Autodesk Inventor part; units mm, degrees
ref_plane "YZ Plane" through (0, 0, 0) normal (1, 0, 0) x (0, 1, 0)
ref_plane "XZ Plane" through (0, 0, 0) normal (0, 1, 0) x (-1, 0, 0)
ref_plane "XY Plane" through (0, 0, 0) normal (0, 0, 1) x (1, 0, 0)
sketch "Sketch1" plane through (0, 0, 0) normal (0, 0, 1) x (1, 0, 0)
  line L0 (-31.45, -31.45) -> (31.45, -31.45)
  line L1 (31.45, -31.45) -> (31.45, 31.45)
  line L2 (31.45, 31.45) -> (-31.45, 31.45)
  line L3 (-31.45, 31.45) -> (-31.45, -31.45)
  line L4 (-31.45, -31.45) -> (31.45, 31.45) construction
  line L5 (31.45, -31.45) -> (-31.45, 31.45) construction
  line L6 (-36.45, 36.45) -> (36.45, 36.45)
  line L7 (36.45, 36.45) -> (36.45, -36.45)
  line L8 (36.45, -36.45) -> (-36.45, -36.45)
  line L9 (-36.45, -36.45) -> (-36.45, 36.45)
  point P0 (0, 0)
  dimension "d0" = 62.9
  dimension "d1" = 62.9
  dimension "d2" = 5
extrude "Extrusion1" add sketch "Sketch1" along normal blind 85
sketch "Sketch2" plane through (0, 0, 0) normal (0, 0, -1) x (-1, 0, 0)
  line L0 (31.45, 31.45) -> (-31.45, 31.45)
  line L1 (31.45, -31.45) -> (-31.45, -31.45)
  line L2 (-31.45, -31.45) -> (-31.45, 31.45)
  line L3 (-31.45, 31.45) -> (31.45, 31.45)
  line L4 (31.45, 31.45) -> (31.45, -31.45)
  line L5 (31.45, -31.45) -> (-31.45, 31.45) construction
  line L6 (-31.45, -31.45) -> (31.45, 31.45) construction
  point P0 (0, 0)
  point P1 (31.45, 31.45)
extrude "Extrusion2" add sketch "Sketch2" against normal blind 12.144
sketch "Sketch3" plane through (-36.45, -36.45, 0) normal (-1, 0, 0) x (0, 0, 1)
  line L0 (85, 0) -> (85, 72.9)
  line L1 (85, 0) -> (0, 0)
  line L2 (0, 0) -> (0, 67.9)
  line L3 (0, 67.9) -> (85, 67.9)
  line L4 (85, 67.9) -> (85, 0)
  point P0 (0, 36.45)
extrude "Extrusion3" cut sketch "Sketch3" against normal blind 5
sketch "Sketch4" plane through (0, 0, 0) normal (0, 0, -1) x (-1, 0, 0)
  point P0 (0, 0)
sketch "Sketch5" plane through (-36.45, 31.45, 0) normal (-1, 0, 0) x (0, 0, 1)
  line L0 (0, 5) -> (0, 0)
  line L1 (0, 5) -> (85, 5)
  line L2 (0, 0) -> (85, 0)
  line L3 (85, 5) -> (85, 0)
  point P0 (0, -31.45)
extrude "Extrusion4" cut sketch "Sketch5" against normal blind 5
sketch "Sketch6" plane through (0, 0, 0) normal (0, 0, -1) x (-1, 0, 0)
  circle A0 centre (0, 0) radius 22.545
  dimension "d11" = 45.09
extrude "Extrusion5" cut sketch "Sketch6" against normal blind 5
sketch "Sketch7" plane through (0, 0, 5) normal (0, 0, -1) x (-1, 0, 0)
  circle A0 centre (0, 0) radius 25.4
  dimension "d14" = 50.8
sketch "Sketch8" plane through (0, 0, 12.144) normal (0, 0, 1) x (1, 0, 0)
  point P0 (0, 0)
extrude "Extrusion6" cut sketch "Sketch7" against normal blind 10
sketch "Sketch12" plane through (36.45, 36.45, 85) normal (0, 1, 0) x (1, 0, 0)
  circle A0 centre (-33.8267, 41.9258) radius 12.7
  point P0 (-36.45, 85)
extrude "Extrusion10" cut sketch "Sketch12" along normal blind 5
sketch "Sketch13" plane through (31.45, -31.45, 85) normal (-1, 0, 0) x (0, 0, 1)
  ellipse E0 centre (-53.33, 18.7291) end of major axis (-50.83, 18.7291) minor radius 2.5
  ellipse E1 centre (-27.93, 44.1291) end of major axis (-25.43, 44.1291) minor radius 2.5
  ellipse E2 centre (-53.33, 44.1291) end of major axis (-50.83, 44.1291) minor radius 2.5
  ellipse E3 centre (-27.93, 18.7291) end of major axis (-25.43, 18.7291) minor radius 2.5
  point P0 (-85, 31.45)
extrude "Extrusion11" cut sketch "Sketch13" against normal blind 5
sketch "Sketch14" plane through (-31.45, -36.45, 0) normal (-1, 0, 0) x (0, 0, 1)
  circle A0 centre (6.072, 70.4) radius 1.5
  line L0 (0, 72.9) -> (85, 72.9)
  line L1 (0, 0) -> (0, 67.9)
  line L2 (12.144, 5) -> (12.144, 67.9)
  circle A1 centre (6.072, 2.5) radius 1.5
  line L3 (85, 0) -> (0, 0)
  circle A2 centre (78.928, 70.4) radius 1.5
  circle A3 centre (78.928, 2.5) radius 1.5
  line L4 (85, 5) -> (85, 0)
  point P0 (0, 36.45)
  dimension "d43" = 3
  dimension "d44" = 2.5
  dimension "d45" = 6.072
  dimension "d46" = 12.144
  dimension "d47" = 3
  dimension "d48" = 2.5
  dimension "d49" = 6.072
  dimension "d50" = 3
  dimension "d51" = 6.072
  dimension "d52" = 2.5
  dimension "d53" = 3
  dimension "d54" = 6.072
extrude "Extrusion12" cut sketch "Sketch14" against normal blind 5
thread "Thread5"
thread "Thread6"
thread "Thread7"
thread "Thread8"
sketch "Sketch15" plane through (36.45, -36.45, 0) normal (0, -1, 0) x (1, 0, 0)
  circle A0 centre (-33.8267, 43.0742) radius 12.7
  circle A1 centre (-33.8267, 43.0742) radius 4.775
  point P0 (-36.45, 0)
  dimension "d65" = 9.55
extrude "Extrusion13" cut sketch "Sketch15" against normal blind 5 contours A1
properties part number "soporte 2.0"
For this review, take the finished solid that the model builds, in its own axes (mm). A direction names the side the tool comes from. Round coordinates to 2 decimals unless told otherwise and drop trailing zeros. Loops run counter-clockwise (first coordinate to the right, second up) from the corner with the lowest first, then second, coordinate; pieces in that order, holes last. Notation, with made-up numbers: (40, 36) - (52, 36) arc R16 cw to (52, 65) - close; hole circle Ø1 at (-36.75, -6). An arc over 180 degrees is marked (long way). One line per item, written item: value. Start each with the question number.
Item 1: For faces 1 (the flat face through (0, 31.45, 48)), 2 (the flat face through (2, 36.45, 42)), 3 (the cylindrical face through (5.506, -24.796, 8.522)), 4 (the cylindrical face through (-28.985, 35.437, 5.877)), 5 (the flat face through (-31.45, -3, 11)), list the 3-axis set-ups (+Z, -Z, +X, -X, +Y, -Y) from which the entire face can be reached by the end or side of a thin tool; tool diameter is ignored.
Item 2: Take a section at A-A (y = 0). Give the boundary of the cut face in (x, z) (3 decimals).
Item 3: Take a section at C-C (x = -19). Give the boundary of the cut face in (y, z), plus the area to 3 significant figures.
Item 4: Take a section at B-B (z = 52.5). Give the boundary of the cut face in (x, y), plus the area to 4 significant figures.
Item 5: The part is to be moulded in two halves that separate along Z. For faces 6 (the flat face through (-26.45, 34, 6)), 7 (the flat face through (36.45, 1, 42)), 8 (the flat face through (10, -21, 5)), say which applies: +Z half, -Z half, draft (parallel to the pull), parting line (faces both ways), or undercut.
Item 6: Take a section at D-D (y = -33.95). Give the boundary of the cut face in (x, z) (3 decimals).
Item 7: Clearance check with flat-ended pins moving along their axes: pin 1 Ø19 at (x, y) = (-5.5, 11.5) entering from +Z; pin 2 Ø2.5 at (y, z) = (33.95, 78.928) entering from -X; pin 3 Ø12 at (y, z) = (17, 55) entering from -X. State where each tip first meets the part, or that it passes through.
Item 8: For L1, parallel to Y at x = 0, z = 3.45 (3 decimals); L2, parallel to Y at x = 9.5, z = 50; L3, parallel to Z at x = -29, y = -33, list the stretches that pass through material, from the lowest coordinate up.
Answer below:
1. face 1: +Z, -X
1. face 2: +Z, -Z, +X, -X, +Y
1. face 3: +Z
1. face 4: -X
1. face 5: +Z, -Z, -X, +Y, -Y
2. outline: (-31.45, 0) - (-22.545, 0) - (-22.545, 5) - (-25.4, 5) - (-25.4, 12.144) - (-31.45, 12.144) - close; (22.545, 0) - (36.45, 0) - (36.45, 85) - (31.45, 85) - (31.45, 12.144) - (25.4, 12.144) - (25.4, 5) - (22.545, 5) - close
3. outline: (-36.45, 0) - (-12.14, 0) - (-12.14, 5) - (-16.86, 5) - (-16.86, 12.14) - (-31.45, 12.14) - (-31.45, 85) - (-36.45, 85) - close; (12.14, 0) - (36.45, 0) - (36.45, 85) - (31.45, 85) - (31.45, 12.14) - (16.86, 12.14) - (16.86, 5) - (12.14, 5) - close
3. area: 1,250 mm2
4. outline: (-31.45, -36.45) - (36.45, -36.45) - (36.45, 36.45) - (-31.45, 36.45) - (-31.45, 31.45) - (31.45, 31.45) - (31.45, -31.45) - (-31.45, -31.45) - close
4. area: 993.5 mm2
5. face 6: undercut
5. face 7: draft
5. face 8: +Z half
6. outline: (-31.45, 0) - (36.45, 0) - (36.45, 85) - (-31.45, 85) - (-31.45, 80.428) - (-26.45, 80.428) - (-26.45, 77.428) - (-31.45, 77.428) - (-31.45, 7.572) - (-26.45, 7.572) - (-26.45, 4.572) - (-31.45, 4.572) - close; hole circle Ø9.55 at (2.623, 43.074)
7. pin 1: passes through
7. pin 2: stops at x = -26.45
7. pin 3: stops at x = 31.45
8. L1: y = -36.45 to -22.545, 22.545 to 36.45
8. L2: y = -36.45 to -31.45, 31.45 to 36.45
8. L3: z = 0 to 4.91, 7.23 to 77.77, 80.09 to 85
